```python
from build123d import *

# Parameters (mm, degrees)
SKETCH_1_W      = 30
SKETCH_1_H      = 14
EXTRUDE_1_DEPTH = 12
FILLET_1_R      = 2


with BuildPart() as part:
    # Эскиз1 → Бобышка-Вытянуть1 (new body)
    with BuildSketch(Plane.XY):
        Rectangle(SKETCH_1_W, SKETCH_1_H)
    extrude(amount=EXTRUDE_1_DEPTH)

    # Эскиз2 → Вырез-Повернуть1 (revolve, cut)
    with BuildSketch(Plane(origin=(0, 7.5, 0), x_dir=(1, 0, 0), z_dir=(0, 1, 0))):
        Polygon((0, 0), (0, -12), (8.1, -12), (8.1, -9.325), (6.1, -9.325), (6.1, -3.825), (8.1, -3.825), (8.1, 0), align=None)
    revolve(axis=Axis((0, 7.5, -4.413755415), (0, 0, 1)), mode=Mode.SUBTRACT)

    # Скругление1
    fillet_1_edges = [part.edges().sort_by_distance(p)[0] for p in [
        (-15, 0, 12),
        (0, -7, 12),
        (-11.542276586, 7, 0),
        (-11.542276586, 7, 12),
        (15, 0, 12),
        (0, -7, 0),
        (-15, 0, 0),
        (11.542276586, 7, 0),
        (15, 0, 0),
        (11.542276586, 7, 12),
        (15, -7, 6),
        (-15, -7, 6),
        (-15, 7, 6),
        (15, 7, 6),
    ]]
    fillet(fillet_1_edges, radius=FILLET_1_R)


solid = part.part
```
Geometry check sheet. Reference: the model listing, model coordinates, mm. A direction names the side the tool comes from. Coordinates: 2 decimals unless noted, no trailing zeros. Loops run counter-clockwise (first coordinate to the right, second up) from the corner with the lowest first, then second, coordinate; pieces in that order, holes last.
Item 1: Sectioned sample at C-C, the plane x = -11.5. Record the boundary of the cut face in (y, z).
Item 2: Access from +Z, -Z, +X, -X, +Y, -Y to the whole of each face (thin tool, end or side, straight path). Record for faces 1 (the face through (-0.17, -0.6, 10.64)), 2 (the face through (-14.43, -6.4, 6.06)), 3 (the face through (0, 1, 3.825)).
Item 3: Go/stop test with flat-tipped pins: pin 1 Ø4 at (x, y) = (1.5, 4.5) entering from -Z; pin 2 Ø2.5 at (x, y) = (0.5, 2.5) entering from +Z (3 decimals); pin 3 Ø2 at (x, z) = (0.5, 5.5) entering from +Y. Record where each tip stops, or that it passes through.
Item 4: Release check for a two-part mould opening along X. For faces 4 (the face through (14.4, 0.07, 11.43)), 5 (the face through (-0.17, -0.6, 1.89)), 6 (the face through (-10, 7, 6)) record: released by +X, released by -X, zero draft, split by the parting line, or undercut.
Item 5: Sectioned sample at B-B, the plane x = 0. Record the boundary of the cut face in (y, z) (3 decimals).
Item 6: Thickness scan on line 1 (X direction, y = 6, z = 1); line 2 (X direction, y = 1.5, z = 0.5); line 3 (Y direction, x = -4.5, z = 3). Record the ranges inside material, lowest first.
Item 7: Sectioned sample at A-A, the plane z = 4.25. Record the boundary of the cut face in (x, y).
Check result:
1. outline: (-7, 2) arc R2 ccw to (-5, 0) - (5, 0) arc R2 ccw to (7, 2) - (7, 10) arc R2 ccw to (5, 12) - (-5, 12) arc R2 ccw to (-7, 10) - close
2. face 1: +Z, +Y
2. face 2: +Z, -Z, -X, -Y
2. face 3: -Z, +Y
3. pin 1: passes through
3. pin 2: stops at z = 9.325
3. pin 3: stops at y = 1.59
4. face 4: released by +X
4. face 5: undercut
4. face 6: zero draft
5. outline: (-7, 2) arc R2 ccw to (-5, 0) - (-0.6, 0) - (-0.6, 3.825) - (1.4, 3.825) - (1.4, 9.325) - (-0.6, 9.325) - (-0.6, 12) - (-5, 12) arc R2 ccw to (-7, 10) - close
6. line 1: x = -14.41 to -7.96, 7.96 to 14.41
6. line 2: x = -14.32 to -5.44, 5.44 to 14.32
6. line 3: y = -7 to 0.77
7. outline: (-15, -5) arc R2 ccw to (-13, -7) - (13, -7) arc R2 ccw to (15, -5) - (15, 5) arc R2 ccw to (13, 7) - (6.08, 7) arc R6.1 cw to (-6.08, 7) - (-13, 7) arc R2 ccw to (-15, 5) - close
